Check sheet for the modelled part. Datum: model origin and axes. Units: mm. Face numbers are marked on the shaded views. A direction names the side the tool comes from. Coordinates: 2 decimals unless noted, no trailing zeros. Loops run counter-clockwise (first coordinate to the right, second up) from the corner with the lowest first, then second, coordinate; pieces in that order, holes last. Notation, with made-up numbers: M 41,-2.5 L 93,-2.5 A18 ccw 93,8.5 Z; hole C 6.5,23.25 d11. An arc over 180 degrees is marked long. Use CSV: the item, a comma, the result in double quotes. Start each with the question number.
(1) Scan lines: line 1 (Z direction, x = 37, y = 0); line 2 (Z direction, x = 44, y = 0); line 3 (X direction, y = -36, z = 73). Record each from-to range of solid material in increasing order.
(2) Go/stop test with flat-tipped pins: pin 1 Ø2 at (x, z) = (60.5, -35.5) entering from -Y; pin 2 Ø1 at (x, y) = (35, 21) entering from +Z; pin 3 Ø1.7 at (x, y) = (45, 35.5) entering from -Z. Record where each tip stops, or that it passes through.
(3) Set-up check for the marked faces 1, 2 and 3: record each of +Z, -Z, +X, -X, +Y, -Y from which the full face is reachable in a straight line by a thin tool's end or side.
(4) Section check A-A on x = 5. Record the cut outline in (y, z), and give its area (3 significant figures).
(5) Section check B-B on x = 22. Record the cut outline in (y, z).
(6) Draft check along Z on the marked faces 4, 5 and 6. Enter one of: pulls with the +Z half, pulls with the -Z half, needs draft (parallel to the pull), parting line crosses it, or undercut.
Autodesk Inventor part; units mm, degrees
ref_plane "РабПлоскость1" through (0, 32.5, 0) normal (0, 1, 0) x (-1, 0, 0)
ref_plane "YZ Plane" through (0, 0, 0) normal (1, 0, 0) x (0, 1, 0)
ref_plane "XY Plane" through (0, 0, 0) normal (0, 0, 1) x (1, 0, 0)
sketch "Эскиз1" plane through (0, 0, 0) normal (0, 0, 1) x (1, 0, 0)
  line L0 (0, 32.5) -> (70, 32.5)
  line L1 (0, 0) -> (109.6934, 0)
  line L2 (0, 32.5) -> (0, 44.804)
  line L3 (35, 68.0113) -> (35, 17.7812) construction
  line L4 (0, 80) -> (70, 80) construction
  line L5 (70, 32.5) -> (0, 32.5)
  line L6 (70, 32.5) -> (70, 44.804)
  line L7 (35, 68.0113) -> (35, 105.8973) construction
  line L8 (35, 90.75) -> (30.3125, 90.75)
  line L9 (30.3125, 90.75) -> (32.3125, 90.75) construction
  line L10 (35, 86.4571) -> (28.75, 86.4571)
  line L11 (30.3125, 90.75) -> (28.75, 86.4571)
  line L12 (28.75, 86.4571) -> (28.75, 75.5)
  line L13 (35, 86.4571) -> (41.25, 86.4571)
  line L14 (39.6875, 90.75) -> (41.25, 86.4571)
  line L15 (41.25, 86.4571) -> (41.25, 75.5)
  line L16 (39.6875, 90.75) -> (35, 90.75)
  line L17 (28.75, 75.5) -> (25.75, 75.5)
  line L18 (25.75, 75.5) -> (25.75, 72.7004)
  line L19 (25.75, 72.7004) -> (25.75, 58.75)
  arc A0 (15.75, 48.75) -> (25.75, 58.75) centre (15.75, 58.75) ccw
  line L20 (35, 90.75) -> (39.6875, 90.75)
  line L21 (35, 86.4571) -> (41.25, 86.4571)
  line L22 (39.6875, 90.75) -> (41.25, 86.4571)
  line L23 (41.25, 86.4571) -> (41.25, 75.5)
  line L24 (44.25, 75.5) -> (44.25, 72.7004)
  line L25 (44.25, 72.7004) -> (44.25, 58.75)
  arc A1 (44.25, 58.75) -> (54.25, 48.75) centre (54.25, 58.75) ccw
  line L26 (44.25, 75.5) -> (41.25, 75.5)
  line L27 (15.75, 48.75) -> (0, 48.75)
  line L28 (0, 48.75) -> (0, 44.804)
  line L29 (54.25, 48.75) -> (70, 48.75)
  line L30 (70, 48.75) -> (70, 43.7446)
  point P0 (0, 46.804)
  point P1 (12.5, 90.75)
  point P2 (57.5, 90.75)
  point P3 (70, 46.804)
  point P4 (57.5, 90.75)
  point P5 (25.75, 42.5)
  dimension "d0" = 65
  dimension "d1" = 70
  dimension "d2" = 160
  dimension "d9" = 45
  dimension "d10" = 70
  dimension "d15" = 2
  dimension "d18" = 2
  dimension "d28" = 4.6875
  dimension "d31" = 6.25
  dimension "d32" = 70
  dimension "d34" = 181.5
  dimension "d35" = 3
  dimension "d36" = 10
ref_plane "РабПлоскость1" through (0, 32.5, 0) normal (0, 1, 0) x (-1, 0, 0)
revolve "Вращение2" add sketch "Эскиз1" angle 360 about axis through (0, 0, 0) along (1, 0, 0)
sketch "Эскиз2" plane through (0, 32.5, 0) normal (0, 1, 0) x (-1, 0, 0)
  line L0 (-70, -8.9471) -> (0, -8.9471)
  line L1 (0, -8.9471) -> (0, 9.0529)
  line L2 (0, 9.0529) -> (-70, 9.0529)
  line L3 (-70, 9.0529) -> (-70, -8.9471)
  line L4 (-70, 32.5) -> (-70, -32.5)
  point P0 (0, 0)
  dimension "d21" = 18
  dimension "d22" = 0
  dimension "d23" = 70
extrude "Выдавливание1" cut sketch "Эскиз2" along normal blind 4.4 and the other way blind 19.45
chamfer "Фаска1" distance 1 angle 45 2 edges at (0, -48.75, 0) (70, -48.75, 0)
equation "\"d17\" = d11"
properties part number "звездочка" material "Сталь, углеродистая"
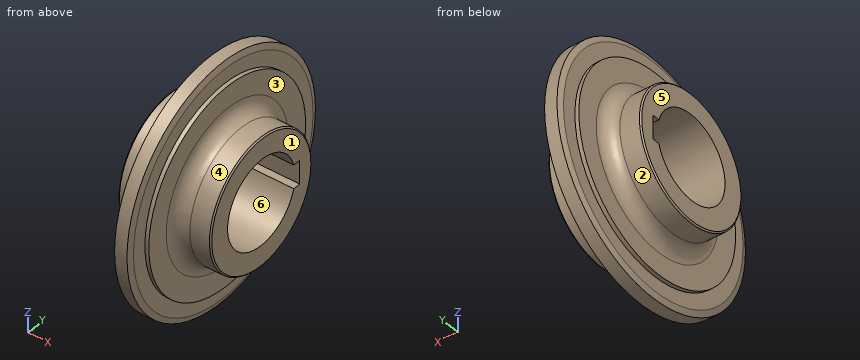
Outcome:
1,line 1,"z = -90.75 to -32.5, 32.5 to 90.75"
1,line 2,"z = -75.5 to -32.5, 32.5 to 75.5"
1,line 3,"x = 28.75 to 41.25"
2,pin 1,"stops at y = -34.44"
2,pin 2,"stops at z = 88.4"
2,pin 3,"stops at z = -66.84"
3,face 1,"+Z, -Z, +X, +Y, -Y"
3,face 2,"-X"
3,face 3,"+X"
4,outline,"C 0,0 d97.5; hole M 31.21,9.05 A32.5 ccw long 31.24,-8.95 L 36.9,-8.95 L 36.9,9.05 Z"
4,area,"4,060 mm²"
5,outline,"C 0,0 d101.89; hole M 31.21,9.05 A32.5 ccw long 31.24,-8.95 L 36.9,-8.95 L 36.9,9.05 Z"
6,face 4,"parting line crosses it"
6,face 5,"needs draft"
6,face 6,"undercut"
